```python
from build123d import *

# Parameters (mm, degrees)
SKETCH1_W           = 2438.4
SKETCH1_H           = 1219.2
BOSS_EXTRUDE1_DEPTH = 9.525
SKETCH2_W           = 88.9
SKETCH2_H           = 76.2
CUT_EXTRUDE1_DEPTH  = 20.05
CHAMFER1_SIZE       = 2.54


with BuildPart() as part:
    # Sketch1 → Boss-Extrude1 (new body, symmetric)
    with BuildSketch(Plane(origin=(0, 0, 0), x_dir=(1, 0, 0), z_dir=(0, 1, 0))):
        with Locations((1219.2, 609.6)):
            Rectangle(SKETCH1_W, SKETCH1_H)
    extrude(amount=BOSS_EXTRUDE1_DEPTH, both=True)

    # Sketch2 → Cut-Extrude1 (cut, through all)
    with BuildSketch(Plane(origin=(0, 9.525, 0), x_dir=(1, 0, 0), z_dir=(0, 1, 0))):
        with Locations((44.45, 1181.1)):
            Rectangle(SKETCH2_W, SKETCH2_H)
        with Locations((690.5625, 1181.1)):
            Rectangle(SKETCH2_W, SKETCH2_H)
        with Locations((1435.1127, 1181.1)):
            Rectangle(SKETCH2_W, SKETCH2_H)
        with Locations((2082.8, 1181.1)):
            Rectangle(SKETCH2_W, SKETCH2_H)
        with Locations((2393.95, 1181.1)):
            Rectangle(SKETCH2_W, SKETCH2_H)
        with Locations((1435.1127, 38.1)):
            Rectangle(SKETCH2_W, SKETCH2_H)
        with Locations((690.5625, 38.1)):
            Rectangle(SKETCH2_W, SKETCH2_H)
        with Locations((2393.95, 38.1)):
            Rectangle(SKETCH2_W, SKETCH2_H)
        with Locations((44.45, 38.1)):
            Rectangle(SKETCH2_W, SKETCH2_H)
    extrude(amount=-CUT_EXTRUDE1_DEPTH, mode=Mode.SUBTRACT)

    # Chamfer1
    chamfer1_edges = [part.edges().sort_by_distance(p)[0] for p in [
        (646.1125, 9.525, -1181.1),
        (690.5625, 9.525, -1143),
        (735.0125, 9.525, -1181.1),
        (44.45, 9.525, -1143),
        (88.9, 9.525, -1181.1),
        (0, 9.525, -609.6),
        (367.50625, 9.525, 0),
        (1062.8376, 9.525, 0),
        (1914.53135, 9.525, 0),
        (2438.4, 9.525, -609.6),
        (2238.375, 9.525, -1219.2),
        (1758.95635, 9.525, -1219.2),
        (1062.8376, 9.525, -1219.2),
        (367.50625, 9.525, -1219.2),
        (1479.5627, 9.525, -38.1),
        (1435.1127, 9.525, -76.2),
        (1390.6627, 9.525, -38.1),
        (735.0125, 9.525, -38.1),
        (690.5625, 9.525, -76.2),
        (646.1125, 9.525, -38.1),
        (2393.95, 9.525, -76.2),
        (2349.5, 9.525, -38.1),
        (88.9, 9.525, -38.1),
        (44.45, 9.525, -76.2),
        (2349.5, 9.525, -1181.1),
        (2393.95, 9.525, -1143),
        (2038.35, 9.525, -1181.1),
        (2082.8, 9.525, -1143),
        (2127.25, 9.525, -1181.1),
        (1479.5627, 9.525, -1181.1),
        (1390.6627, 9.525, -1181.1),
        (1435.1127, 9.525, -1143),
    ]]
    chamfer(chamfer1_edges, length=CHAMFER1_SIZE)


solid = part.part
```
Geometry check sheet. Reference: the model listing, model coordinates, mm. Coordinates: 2 decimals unless noted, no trailing zeros. Loops run counter-clockwise (first coordinate to the right, second up) from the corner with the lowest first, then second, coordinate; pieces in that order, holes last. Notation, with made-up numbers: (78.25, 53.25) -> (112.25, 53.25) arc R33 ccw to (112.25, 91.25) -> close; hole circle Ø11 at (76, 84.5). An arc over 180 degrees is marked (long way). Put each result on its own line as item: value.
1) Cross-section at C-C on x = 677.5. Record the boundary of the cut face in (y, z) (3 decimals), plus the area to 3 significant figures.
Result set:
outline: (-9.525, -1143) -> (6.985, -1143) -> (9.525, -1140.46) -> (9.525, -78.74) -> (6.985, -76.2) -> (-9.525, -76.2) -> close
area: 20,300 mm^2
2) Gauge pin test, flat ends, axial feed: pin 1 Ø8.5 at (x, y) = (1415, -3.5) entering from +Z; pin 2 Ø5 at (y, z) = (-1.5, -1191.5) entering from -X; pin 3 Ø8.5 at (x, y) = (26, -4.5) entering from -Z. Record the tip position at first contact, or that the pin passes through.
Result set:
pin 1: stops at z = -76.2
pin 2: stops at x = 88.9
pin 3: stops at z = -1143
3) Cross-section at B-B on x = 2088. Record the boundary of the cut face in (y, z) (3 decimals), plus the area to 3 significant figures.
Result set:
outline: (-9.525, -1143) -> (6.985, -1143) -> (9.525, -1140.46) -> (9.525, -2.54) -> (6.985, 0) -> (-9.525, 0) -> close
area: 21,800 mm^2
4) Thickness scan on line 1 (X direction, y = 4.75, z = -60); line 2 (X direction, y = 7.25, z = -327.5) (3 decimals); line 3 (Z direction, x = 1815, y = 7.5) (3 decimals). Record the ranges inside material, lowest first.
Result set:
line 1: x = 88.9 to 646.11, 735.01 to 1390.66, 1479.56 to 2349.5
line 2: x = 0.265 to 2438.135
line 3: z = -1218.685 to -0.515
